Input: dimensioned drawing with shaded views. Units: mm. Origin: part minimum x, y, z. A direction names the side the tool comes from. Round coordinates to 2 decimals unless told otherwise and drop trailing zeros. Order: outer loops, then holes, each group sorted by start corner. A loop starts at its lowest first (then second) coordinate and runs counter-clockwise, first axis right, second up.
Item 1: Line query: L1, parallel to Y at x = 48.5, z = 3; L2, parallel to Y at x = 48.4, z = 36.5; L3, parallel to Y at x = 20, z = 41.5. Output: solid intervals per line, ascending.
Item 2: Mould query, pull axis X, two halves, no side actions, for the marked faces 3, 4 and 5. Classes: released by +X, released by -X, zero draft, split by the parting line, or undercut.
Item 3: Cut plane D-D on z = 36.5. Output: boundary loops of the cut face in (x, y), then the cut area to 3 significant figures.
Item 4: Reachability of the marked faces 1 and 2 from +Z, -Z, +X, -X, +Y, -Y: full face, straight path, thin tool, end or side. Return the list, or none.
Item 5: Cut plane A-A on x = 10. Output: boundary loops of the cut face in (y, z), then the cut area to 3 significant figures.
Item 6: First-contact query: pin 1 (1.2 mm diameter, centred on x = 40, z = 3, fed in from +Y). Flat tip, straight axial feed; report the tip coordinate or a pass-through.
Item 7: Cut plane B-B on y = 16. Output: boundary loops of the cut face in (x, z).
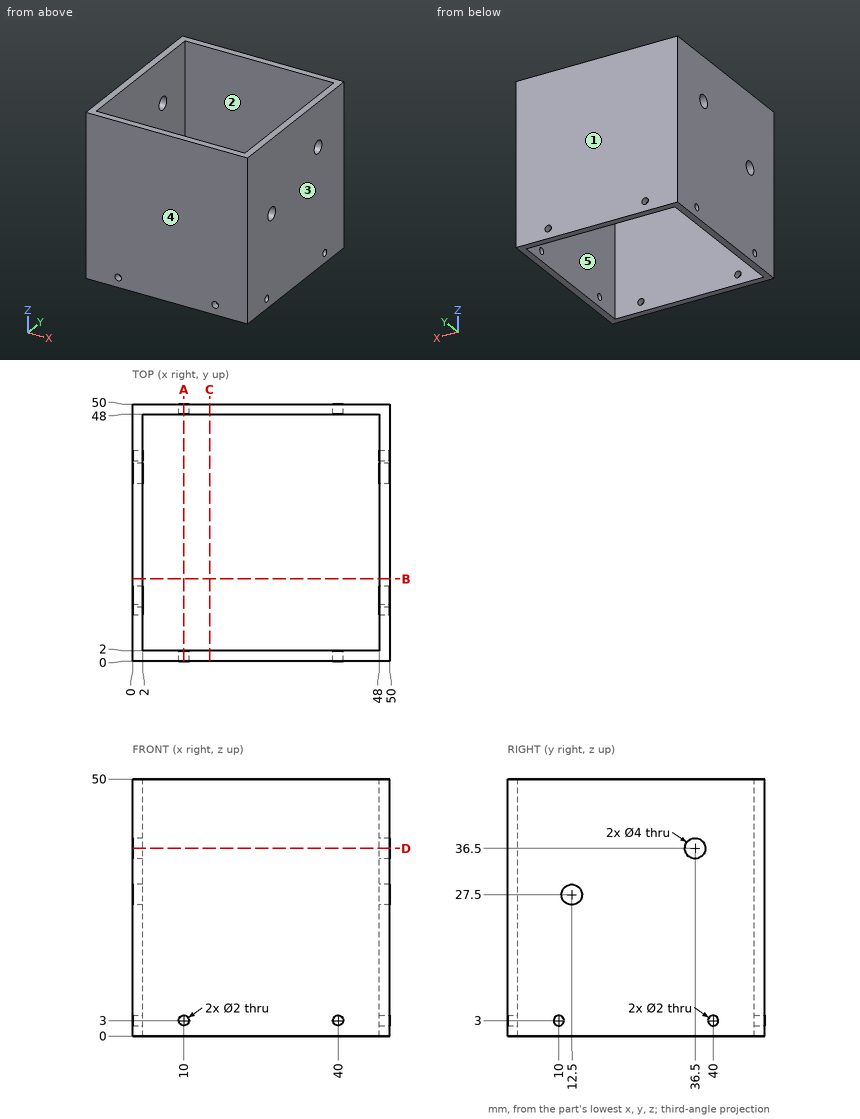
From the geometry:
1. L1: y = 0 to 9, 11 to 39, 41 to 50
1. L2: y = 0 to 34.5, 38.5 to 50
1. L3: y = 0 to 2, 48 to 50
2. face 3: released by +X
2. face 4: zero draft
2. face 5: undercut
3. outline: (0, 0) - (50, 0) - (50, 34.5) - (48, 34.5) - (48, 2) - (2, 2) - (2, 34.5) - (0, 34.5) - close; (0, 38.5) - (2, 38.5) - (2, 48) - (48, 48) - (48, 38.5) - (50, 38.5) - (50, 50) - (0, 50) - close
3. area: 368 mm2
4. face 1: +Z, -Z, +X, -X, +Y
4. face 2: +Z, -Z
5. outline: (0, 0) - (2, 0) - (2, 2) - (0, 2) - close; (0, 4) - (2, 4) - (2, 50) - (0, 50) - close; (48, 0) - (50, 0) - (50, 2) - (48, 2) - close; (48, 4) - (50, 4) - (50, 50) - (48, 50) - close
5. area: 192 mm2
6. pin 1: passes through
7. outline: (0, 0) - (2, 0) - (2, 50) - (0, 50) - close; (48, 0) - (50, 0) - (50, 50) - (48, 50) - close
